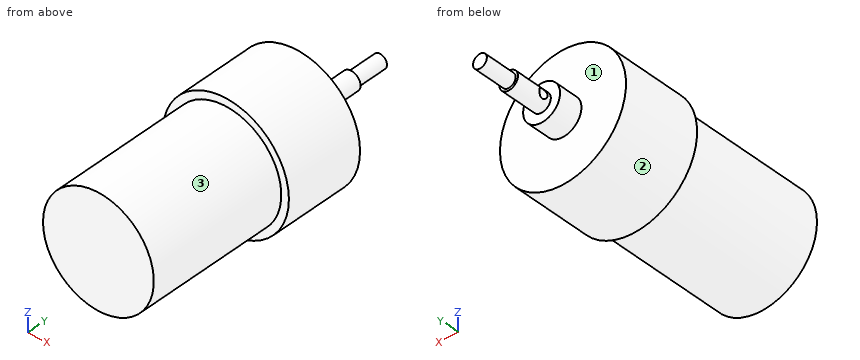
Autodesk Inventor part; units mm, degrees
ref_plane "YZ Plane" through (0, 0, 0) normal (1, 0, 0) x (0, 1, 0)
ref_plane "XZ Plane" through (0, 0, 0) normal (0, 1, 0) x (-1, 0, 0)
ref_plane "XY Plane" through (0, 0, 0) normal (0, 0, 1) x (1, 0, 0)
sketch "スケッチ8" plane through (0, 0, 0) normal (0, 1, 0) x (-1, 0, 0)
  circle A0 centre (0, 0) radius 12
  dimension "d29" = 24
extrude "押し出し6" add sketch "スケッチ8" along normal blind 31
ref_plane "作業平面4" through (0, 31, 0) normal (0, 1, 0) x (1, 0, 0)
sketch "スケッチ9" plane through (0, 31, 0) normal (0, 1, 0) x (1, 0, 0)
  circle A0 centre (0, 0) radius 13.65
  dimension "d33" = 27.3
extrude "押し出し7" add sketch "スケッチ9" along normal blind 17.3
ref_plane "作業平面5" through (0, 48.3, 0) normal (0, 1, 0) x (1, 0, 0)
sketch "スケッチ10" plane through (0, 48.3, 0) normal (0, 1, 0) x (1, 0, 0)
  circle A0 centre (0, 0) radius 4
  dimension "d37" = 8
extrude "押し出し8" add sketch "スケッチ10" along normal blind 5.2
ref_plane "作業平面6" through (0, 53.5, 0) normal (0, 1, 0) x (1, 0, 0)
sketch "スケッチ11" plane through (0, 53.5, 0) normal (0, 1, 0) x (1, 0, 0)
  circle A0 centre (0, 0) radius 2
  dimension "d41" = 4
extrude "押し出し9" add sketch "スケッチ11" along normal blind 8
ref_plane "作業平面7" through (0, 61.5, 0) normal (0, 1, 0) x (1, 0, 0)
sketch "スケッチ12" plane through (0, 61.5, 0) normal (0, 1, 0) x (1, 0, 0)
  circle A0 centre (0, 0) radius 1.5
  dimension "d45" = 3
extrude "押し出し10" add sketch "スケッチ12" along normal blind 7
sketch "スケッチ13" plane through (0, 61.5, 0) normal (0, 1, 0) x (1, 0, 0)
  circle A0 centre (0, 0) radius 2
  point P0 (2, 0)
ref_plane "作業平面8" through (2, 61.5, 0) normal (1, 0, 0) x (0, 1, 0)
sketch "スケッチ14" plane through (2, 61.5, 0) normal (1, 0, 0) x (0, 1, 0)
  circle A0 centre (-6.2, 0) radius 1
  line L0 (0, -2) -> (0, 2)
  point P0 (-61.5, 0)
  dimension "d48" = 2
  dimension "d49" = 6.2
hole "穴2" at (2, 55.3, 0) direction (-1, 0, 0) diameter 2 end through all
properties part number "daisen_motor"
Source: CAD feature listing. Evaluate the final solid. Frame: model axes, mm. Face numbers are marked on the shaded views. A direction names the side the tool comes from. Round coordinates to 2 decimals unless told otherwise and drop trailing zeros. Loops run counter-clockwise (first coordinate to the right, second up) from the corner with the lowest first, then second, coordinate; pieces in that order, holes last.
(1) Section query A-A (z = 0). Output: boundary loops of the cut face in (x, y), and give its area (3 significant figures).
From the geometry:
outline: (-13.65, 31) - (-12, 31) - (-12, 0) - (12, 0) - (12, 31) - (13.65, 31) - (13.65, 48.3) - (4, 48.3) - (4, 53.5) - (2, 53.5) - (2, 54.3) - (-2, 54.3) - (-2, 53.5) - (-4, 53.5) - (-4, 48.3) - (-13.65, 48.3) - close; (-2, 56.3) - (2, 56.3) - (2, 61.5) - (1.5, 61.5) - (1.5, 68.5) - (-1.5, 68.5) - (-1.5, 61.5) - (-2, 61.5) - close
area: 1,300 mm2
(2) Section query B-B (x = 0). Output: boundary loops of the cut face in (y, z), and give its area (3 significant figures).
From the geometry:
outline: (0, -12) - (31, -12) - (31, -13.65) - (48.3, -13.65) - (48.3, -4) - (53.5, -4) - (53.5, -2) - (61.5, -2) - (61.5, -1.5) - (68.5, -1.5) - (68.5, 1.5) - (61.5, 1.5) - (61.5, 2) - (53.5, 2) - (53.5, 4) - (48.3, 4) - (48.3, 13.65) - (31, 13.65) - (31, 12) - (0, 12) - close; hole circle Ø2 at (55.3, 0)
area: 1,310 mm2
(3) Contact query for flat-ended pins moving along their axis: pin 1 Ø4 at (y, z) = (60.5, 0.5) entering from -X; pin 2 Ø1.2 at (y, z) = (55.3, 0) entering from -X; pin 3 Ø12 at (y, z) = (34, -8.5) entering from +X; pin 4 Ø5 at (x, y) = (3, 49.5) entering from -Z. Output: stop coordinate, or through.
From the geometry:
pin 1: stops at x = -2
pin 2: passes through
pin 3: stops at x = 13.42
pin 4: stops at z = -13.63
(4) Access query for the marked faces 1, 2 and 3. Directions: +Z, -Z, +X, -X, +Y, -Y. A direction counts if a zero-diameter tool reaches every point of the face in a straight line with its end or side. Return the directions, or none.
From the geometry:
face 1: +Y
face 2: +Y, -Y
face 3: -Y
(5) Section query C-C (y = 55.3). Output: boundary loops of the cut face in (x, z), and give its area (3 significant figures).
From the geometry:
outline: (-1.73, -1) arc R2 ccw to (1.73, -1) - close; (-1.73, 1) - (1.73, 1) arc R2 ccw to start
area: 4.91 mm2
(6) Section query D-D (x = -7). Output: boundary loops of the cut face in (y, z).
From the geometry:
outline: (0, -9.75) - (31, -9.75) - (31, -11.72) - (48.3, -11.72) - (48.3, 11.72) - (31, 11.72) - (31, 9.75) - (0, 9.75) - close
(7) Material intervals for probe 1 along Y at (x, z) = (0.6, 0); probe 2 along Z at (x, y) = (-0.1, 55.3); probe 3 along Z at (x, y) = (0, 52), sorted ascending.
From the geometry:
probe 1: y = 0 to 54.3, 56.3 to 68.5
probe 2: z = -2 to -1, 1 to 2
probe 3: z = -4 to 4
